Work out the finished part from the listing and answer in its coordinate system (mm). A direction names the side the tool comes from. Coordinates: 2 decimals unless noted, no trailing zeros. Write each loop counter-clockwise with the first axis right and the second up, starting at its lowest first coordinate (ties: lowest second). Pieces come first, ordered by that corner, then holes. Notation, with made-up numbers: (10, 11) - (49, 11) arc R14 cw to (49, 21) - close; hole circle Ø9 at (36.5, 59.25). An arc over 180 degrees is marked (long way). Use a Markdown table: item, result. Add a question column.
(1) A tool of negligible diameter and unlimited length cuts with its end or side. For faces 5 (the face through (13, 2, -10)), 6 (the face through (14.3, 5, -2.4)), 7 (the face through (-11, 2, 10)), 8 (the face through (-11, 2, -10)), 9 (the face through (13, 2, 10)), from which of +Z, -Z, +X, -X, +Y, -Y can it reach the whole face along a straight path? Write none if from no direction.
(2) The part is cut by section C-C, the plane x = 12.5. Give the vertices of the cut face in (y, z).
(3) The part is cut by section B-B, the plane z = -15. Give the vertices of the cut face in (x, y), then the cut area to 3 significant figures.
(4) For a pull along Y with two mould halves and no side action, classify faces 1 (the face through (1.803, 9.726, 13.331)), 2 (the face through (20, 2, 0)), 3 (the face through (1.803, 2.465, -14.93)), 4 (the face through (1.803, 8.53, -16.617)) as released by +Y, released by -Y, zero draft, split by the parting line, or undercut.
(5) Given pin 1 Ø4 at (y, z) = (3.5, 15) entering from +X; pin 2 Ø1.5 at (x, y) = (16, 2) entering from -Z; pin 3 Ø4 at (x, y) = (-2.5, 7) entering from -Z; pin 4 Ø4 at (x, y) = (9.5, 2) entering from +Z, each flat-ended and moving along its own axis, determine where each tip first touches the part or whether it passes through.
(6) The part is cut by section D-D, the plane y = 9.2. Give the vertices of the cut face in (x, z).
(7) The part is cut by section A-A, the plane y = 1. Give the vertices of the cut face in (x, z).
(8) Find the intervals of material crossed by line 1 (X direction, y = 3.8, z = 0); line 2 (Z direction, x = 2, y = 9); line 3 (Y direction, x = 18.5, z = 0.5), in increasing order. Write a range as from..to.
from build123d import *

# Parameters (mm, degrees)
SKETCH_1_W          = 40
SKETCH_1_H          = 20
SKETCH_1_R          = 2.5
EXTRUDE_1_DEPTH     = 5
SKETCH_2_W          = 7.5
SKETCH_2_H          = 40
EXTRUDE_2_DEPTH     = 10
SKETCH_3_R          = 1.75
CUT_EXTRUDE_1_DEPTH = 10
EXTRUDE_3_DEPTH     = 7.5


with BuildPart() as part:
    # 草图1 → 凸台-拉伸1 (new body)
    with BuildSketch(Plane(origin=(0, 0, 0), x_dir=(1, 0, 0), z_dir=(0, 1, 0))):
        Rectangle(SKETCH_1_W, SKETCH_1_H)
        with Locations(Location((-12.5, 0, 0), (0, 0, 270))):
            Circle(SKETCH_1_R, mode=Mode.SUBTRACT)
        with Locations(Location((12.5, 0, 0), (0, 0, 270))):
            Circle(SKETCH_1_R, mode=Mode.SUBTRACT)
    extrude(amount=EXTRUDE_1_DEPTH)

    # 草图2 → 凸台-拉伸2 (add)
    with BuildSketch(Plane(origin=(0, 5, 0), x_dir=(1, 0, 0), z_dir=(0, 1, 0))):
        with Locations((1.75, 0)):
            Rectangle(SKETCH_2_W, SKETCH_2_H)
    extrude(amount=EXTRUDE_2_DEPTH)

    # 草图3 → 切除-拉伸1 (cut)
    with BuildSketch(Plane(origin=(5.5, 0, 0), x_dir=(0, 0, -1), z_dir=(1, 0, 0))):
        with Locations((-15, 9.2)):
            Circle(SKETCH_3_R)
        with Locations((15, 9.2)):
            Circle(SKETCH_3_R)
    extrude(amount=-CUT_EXTRUDE_1_DEPTH, mode=Mode.SUBTRACT)

    # 草图4 → 凸台-拉伸3 (add)
    with BuildSketch(Plane(origin=(5.5, 0, 0), x_dir=(0, 0, -1), z_dir=(1, 0, 0))):
        Polygon((-20, 5), (-10, 0), (-10, 5), align=None)
        Polygon((10, 5), (10, 0), (20, 5), align=None)
    extrude(amount=-EXTRUDE_3_DEPTH)


solid = part.part
Model answer:
| question | item | result |
|---|---|---|
| 1 | face 5 | -Z, +X, +Y, -Y |
| 1 | face 6 | +Z, -Z, +X, +Y |
| 1 | face 7 | +Z, -X, +Y, -Y |
| 1 | face 8 | -Z, -X, +Y, -Y |
| 1 | face 9 | +Z, +X, +Y, -Y |
| 2 | outline | (0, -10) - (5, -10) - (5, -2.5) - (0, -2.5) - close; (0, 2.5) - (5, 2.5) - (5, 10) - (0, 10) - close |
| 3 | outline | (-2, 2.5) - (5.5, 2.5) - (5.5, 7.45) - (-2, 7.45) - close; (-2, 10.95) - (5.5, 10.95) - (5.5, 15) - (-2, 15) - close |
| 3 | area | 67.5 mm^2 |
| 4 | face 1 | undercut |
| 4 | face 2 | zero draft |
| 4 | face 3 | released by -Y |
| 4 | face 4 | undercut |
| 5 | pin 1 | x = 5.5 |
| 5 | pin 2 | z = -10 |
| 5 | pin 3 | z = -20 |
| 5 | pin 4 | z = 10 |
| 6 | outline | (-2, -20) - (5.5, -20) - (5.5, -16.75) - (-2, -16.75) - close; (-2, -13.25) - (5.5, -13.25) - (5.5, 13.25) - (-2, 13.25) - close; (-2, 16.75) - (5.5, 16.75) - (5.5, 20) - (-2, 20) - close |
| 7 | outline | (-20, -10) - (-2, -10) - (-2, -12) - (5.5, -12) - (5.5, -10) - (20, -10) - (20, 10) - (5.5, 10) - (5.5, 12) - (-2, 12) - (-2, 10) - (-20, 10) - close; hole circle Ø5 at (-12.5, 0); hole circle Ø5 at (12.5, 0) |
| 8 | line 1 | -20..-15, -10..10, 15..20 |
| 8 | line 2 | -20..-16.74, -13.26..13.26, 16.74..20 |
| 8 | line 3 | 0..5 |
